from build123d import *

# Parameters (mm, degrees)
SKETCH2_W           = 70
SKETCH2_H           = 35
BOSS_EXTRUDE1_DEPTH = 35
SKETCH3_W           = 30
SKETCH3_H           = 25
CUT_EXTRUDE1_DEPTH  = 25
SKETCH4_W           = 30
SKETCH4_H           = 25
CUT_EXTRUDE2_DEPTH  = 25
CUT_EXTRUDE3_DEPTH  = 25
CUT_EXTRUDE4_DEPTH  = 25
CUT_EXTRUDE5_DEPTH  = 25
SKETCH8_R           = 5
CUT_EXTRUDE6_DEPTH  = 11
SKETCH9_R           = 5
CUT_EXTRUDE7_DEPTH  = 11


with BuildPart() as part:
    # Sketch2 → Boss-Extrude1 (new body)
    with BuildSketch(Plane(origin=(0, 0, 0), x_dir=(1, 0, 0), z_dir=(0, 1, 0))):
        with Locations((35, 17.5)):
            Rectangle(SKETCH2_W, SKETCH2_H)
    extrude(amount=BOSS_EXTRUDE1_DEPTH)

    # Sketch3 → Cut-Extrude1 (cut)
    with BuildSketch(Plane.XY):
        with Locations((55, 22.5)):
            Rectangle(SKETCH3_W, SKETCH3_H)
    extrude(amount=-CUT_EXTRUDE1_DEPTH, mode=Mode.SUBTRACT)

    # Sketch4 → Cut-Extrude2 (cut)
    with BuildSketch(Plane.XY):
        with Locations((15, 22.5)):
            Rectangle(SKETCH4_W, SKETCH4_H)
    extrude(amount=-CUT_EXTRUDE2_DEPTH, mode=Mode.SUBTRACT)

    # Sketch5 → Cut-Extrude3 (cut)
    with BuildSketch(Plane(origin=(40, 0, 0), x_dir=(0, 0, -1), z_dir=(1, 0, 0))):
        Polygon((0, 10), (25, 35), (0, 35), align=None)
    extrude(amount=-CUT_EXTRUDE3_DEPTH, mode=Mode.SUBTRACT)

    # Sketch6 → Cut-Extrude4 (cut)
    with BuildSketch(Plane.XY.offset(-25)):
        Polygon((70, 35), (70, 20), (55, 35), align=None)
    extrude(amount=-CUT_EXTRUDE4_DEPTH, mode=Mode.SUBTRACT)

    # Sketch7 → Cut-Extrude5 (cut)
    with BuildSketch(Plane.XY.offset(-25)):
        Polygon((0, 35), (0, 20), (15, 35), align=None)
    extrude(amount=-CUT_EXTRUDE5_DEPTH, mode=Mode.SUBTRACT)

    # Sketch8 → Cut-Extrude6 (cut, through all)
    with BuildSketch(Plane(origin=(0, 10, 0), x_dir=(1, 0, 0), z_dir=(0, 1, 0))):
        with Locations((55, 10)):
            Circle(SKETCH8_R)
    extrude(amount=-CUT_EXTRUDE6_DEPTH, mode=Mode.SUBTRACT)

    # Sketch9 → Cut-Extrude7 (cut, through all)
    with BuildSketch(Plane(origin=(0, 10, 0), x_dir=(1, 0, 0), z_dir=(0, 1, 0))):
        with Locations((15, 10)):
            Circle(SKETCH9_R)
    extrude(amount=-CUT_EXTRUDE7_DEPTH, mode=Mode.SUBTRACT)


solid = part.part
Model file for the job. Use its own axes, mm. A direction names the side the tool comes from. Give positions to 0.01 mm unless a question says otherwise; leave off trailing zeros. Loops run counter-clockwise (first coordinate to the right, second up) from the corner with the lowest first, then second, coordinate; pieces in that order, holes last. Notation, with made-up numbers: (16, 77.25) -> (70, 77.25) arc R8 ccw to (70, 87.25) -> close; hole circle Ø1 at (-17, -1.5). An arc over 180 degrees is marked (long way). Use a Markdown table: item, result. Add a question column.
(1) Slice it at B-B on z = -20. List the corners of the cut face in (x, y).
(2) Wall check: line 1 along X through (y, z) = (3.5, -10); line 2 along Z through (x, y) = (15, 4); line 3 along X through (y, z) = (3, -14). Give the ranges that are in metal, low to high.
(3) Slice it at A-A on z = -10. List the corners of the cut face in (x, y).
(4) Tool access for faces 5 (the flat face through (30, 17, -18)), 6 (the flat face through (51, 23, -25)), 7 (the flat face through (7, 27, -30)): list every direction of +Z, -Z, +X, -X, +Y, -Y with a clear straight run to the whole face (end or side of a thin tool).
(5) Mould opens along X. For faces 1 (the cylindrical face through (51, 5, -13)), 2 (the flat face through (35, 17, -35)), 3 (the flat face through (63, 27, -30)), 4 (the cylindrical face through (19.77, 5.07, -11.5)) say: +X half, -X half, draft (parallel to the pull), parting line (faces both ways), or undercut.
(6) Slice it at C-C on y = 23. List the corners of the cut face in (x, z), and give its area (3 significant figures).
(7) Slice it at D-D on x = 31. List the corners of the cut face in (y, z).
(8) Drop flat-ended pins along their axis: pin 1 Ø12.5 at (x, z) = (51, -16.5) entering from +Y; pin 2 Ø10 at (x, z) = (26.5, -8) entering from -Y; pin 3 Ø7.5 at (x, y) = (15, 17) entering from +Z; pin 4 Ø12 at (x, z) = (35, -6.5) entering from +Y. Give the stop position or say it passes through.
Filled sheet:
| question | item | result |
|---|---|---|
| 1 | outline | (0, 0) -> (70, 0) -> (70, 10) -> (40, 10) -> (40, 30) -> (30, 30) -> (30, 10) -> (0, 10) -> close |
| 2 | line 1 | 0 to 10, 20 to 50, 60 to 70 |
| 2 | line 2 | -35 to -15, -5 to 0 |
| 2 | line 3 | 0 to 12, 18 to 52, 58 to 70 |
| 3 | outline | (0, 0) -> (10, 0) -> (10, 10) -> (0, 10) -> close; (20, 0) -> (50, 0) -> (50, 10) -> (40, 10) -> (40, 20) -> (30, 20) -> (30, 10) -> (20, 10) -> close; (60, 0) -> (70, 0) -> (70, 10) -> (60, 10) -> close |
| 4 | face 5 | +Z, -X, +Y |
| 4 | face 6 | +Z, +X, +Y |
| 4 | face 7 | +Z, -Z, -X, +Y |
| 5 | face 1 | undercut |
| 5 | face 2 | draft |
| 5 | face 3 | +X half |
| 5 | face 4 | undercut |
| 6 | outline | (3, -35) -> (67, -35) -> (67, -25) -> (40, -25) -> (40, -13) -> (30, -13) -> (30, -25) -> (3, -25) -> close |
| 6 | area | 760 mm2 |
| 7 | outline | (0, -35) -> (35, -35) -> (35, -25) -> (10, 0) -> (0, 0) -> close |
| 8 | pin 1 | y = 10 |
| 8 | pin 2 | y = 0 |
| 8 | pin 3 | z = -25 |
| 8 | pin 4 | y = 22.5 |
